```python
from build123d import *

# Parameters (mm, degrees)
BODY_DEPTH                     = 8
M3_CLEARANCE_SLOT1_DEPTH       = 8
LPATTERN3_COUNT                = 2
LPATTERN3_PITCH                = 31
LPATTERN3_COUNT_DIR2           = 2
LPATTERN3_PITCH_DIR2           = 31
CUT_EXTRUDE1_DEPTH             = 207.067949958
M3X0_5_TAPPED_HOLE1_D          = 2.5
LPATTERN2_COUNT                = 4
LPATTERN2_PITCH                = 25
CBORE_FOR_M5_SHCS1_D           = 5.5
CBORE_FOR_M5_SHCS1_CBORE_D     = 10
CBORE_FOR_M5_SHCS1_CBORE_DEPTH = 5
M3X0_5_TAPPED_HOLE2_D          = 2.5
M3X0_5_TAPPED_HOLE2_DEPTH      = 6.748924226
M3X0_5_TAPPED_HOLE2_TIP        = 0.751075774
SKETCH22_R                     = 2.5
CUT_EXTRUDE2_DEPTH             = 207.067949958


# Read off the part's stored shape, not the designer's step: M3 Clearance Slot1
with BuildPart() as part:
    # Sketch1 → BODY (new body)
    with BuildSketch(Plane.XY):
        with BuildLine():
            Line((-180, 100), (0, 100))
            Line((0, 100), (0, 0))
            Line((0, 0), (-50, 0))
            Line((-50, 0), (-50, 30))
            ThreePointArc((-50, 30), (-52.928932188, 37.071067812), (-60, 40))
            Line((-60, 40), (-180, 40))
            Line((-180, 40), (-180, 100))
        make_face()
    extrude(amount=BODY_DEPTH)

    # M3 Clearance Slot1 outline → M3 Clearance Slot1 (cut)
    with BuildSketch(Plane.XY):
        with BuildLine():
            Line((-42.3, 92.3), (-37.7, 92.3))
            ThreePointArc((-37.7, 92.3), (-36, 94), (-37.7, 95.7))
            Line((-37.7, 95.7), (-42.3, 95.7))
            ThreePointArc((-42.3, 95.7), (-44, 94), (-42.3, 92.3))
        make_face()
    m3_clearance_slot1 = extrude(amount=M3_CLEARANCE_SLOT1_DEPTH, mode=Mode.SUBTRACT)

    # LPattern3: M3 Clearance Slot1 2 × 2
    with Locations(*[(i * LPATTERN3_PITCH, -j * LPATTERN3_PITCH_DIR2, 0) for i in range(LPATTERN3_COUNT) for j in range(LPATTERN3_COUNT_DIR2) if (i, j) != (0, 0)]):
        add(m3_clearance_slot1, mode=Mode.SUBTRACT)

    # Sketch21 → Cut-Extrude1 (cut, through all)
    with BuildSketch(Plane.XY.offset(8)):
        with BuildLine():
            Line((-27, 89.5), (-22, 89.5))
            ThreePointArc((-22, 89.5), (-11, 78.5), (-22, 67.5))
            Line((-22, 67.5), (-27, 67.5))
            ThreePointArc((-27, 67.5), (-38, 78.5), (-27, 89.5))
        make_face()
    extrude(amount=-CUT_EXTRUDE1_DEPTH, mode=Mode.SUBTRACT)

    # M3x0.5 Tapped Hole1 (through all)
    with Locations(Plane.XY.offset(8)):
        with Locations((-70, 48)):
            m3x0_5_tapped_hole1 = Hole(M3X0_5_TAPPED_HOLE1_D / 2)

    # LPattern2: M3x0.5 Tapped Hole1 ×4
    with Locations(*[(-i * LPATTERN2_PITCH, 0, 0) for i in range(1, LPATTERN2_COUNT)]):
        add(m3x0_5_tapped_hole1, mode=Mode.SUBTRACT)

    # CBORE for M5 SHCS1 (through all)
    with Locations(Plane(origin=(0, 0, 0), x_dir=(-1, 0, 0), z_dir=(0, 0, -1))):
        with Locations((10, 6), (40, 6)):
            CounterBoreHole(CBORE_FOR_M5_SHCS1_D / 2, CBORE_FOR_M5_SHCS1_CBORE_D / 2, CBORE_FOR_M5_SHCS1_CBORE_DEPTH)

    # M3x0.5 Tapped Hole2
    with Locations(Plane.ZY.offset(180)):
        with Locations((4, 82), (4, 76)):
            Hole(M3X0_5_TAPPED_HOLE2_D / 2, depth=M3X0_5_TAPPED_HOLE2_DEPTH)
            with Locations((0, 0, -(M3X0_5_TAPPED_HOLE2_DEPTH + M3X0_5_TAPPED_HOLE2_TIP / 2))):  # 118° drill point
                Cone(0, M3X0_5_TAPPED_HOLE2_D / 2, M3X0_5_TAPPED_HOLE2_TIP, mode=Mode.SUBTRACT)

    # Sketch22 → Cut-Extrude2 (cut, through all)
    with BuildSketch(Plane.XY.offset(8)):
        with Locations((-170, 78.5)):
            Circle(SKETCH22_R)
    extrude(amount=-CUT_EXTRUDE2_DEPTH, mode=Mode.SUBTRACT)


solid = part.part
```
The model under review builds one solid part; all positions refer to its coordinate system, in mm. A direction names the side the tool comes from. Coordinates: 2 decimals unless noted, no trailing zeros. Write each loop counter-clockwise with the first axis right and the second up, starting at its lowest first coordinate (ties: lowest second). Pieces come first, ordered by that corner, then holes. Notation, with made-up numbers: (-13, -26) - (44, -26) arc R9 cw to (44, -15) - close; hole circle Ø4 at (-27, 28.25). An arc over 180 degrees is marked (long way). Answer in a Markdown table with one row per item. Add a question column.
Q1. To check wall thickness, follow line 1 along Y through (x, z) = (-170, 4.25); line 2 along Y through (x, z) = (-40, 3.15); line 3 along Y through (x, z) = (-43.5, 6.5). State the ranges of each line that lie inside material, in increasing order. Write a range as from..to.
Q2. Consider section A-A on y = 70. Give the boundary of the cut face in (x, z), then the cut area to 3 significant figures.
Q3. Draft analysis for pull direction Y (two halves, no side actions). For faces 1 (the face through (-119, 40, 4)), 2 (the face through (-89, 62, 0)), 3 (the face through (-40, 95.7, 4)), 4 (the face through (-5, 63, 4)), state which applies: +Y half, -Y half, draft (parallel to the pull), parting line (faces both ways), or undercut.
Q4. For faces 5 (the face through (-14.619, 4.085, 2.465)), 6 (the face through (-50, 15, 4)), 7 (the face through (-36, 94, 4)), list the 3-axis set-ups (+Z, -Z, +X, -X, +Y, -Y) from which the entire face can be reached by the end or side of a thin tool; tool diameter is ignored.
Q5. Clearance check with flat-ended pins moving along their axes: pin 1 (1.4 mm diameter, centred on x = -39.5, z = 5.5, fed in from -Y); pin 2 (2.5 mm diameter, centred on x = -138, z = 3.5, fed in from -Y); pin 3 (1.5 mm diameter, centred on x = -70, y = 48, fed in from +Z). State where each tip first meets the part, or that it passes through.
Q6. Consider section B-B on x = -128. Give the boundary of the cut face in (y, z), then the cut area to 3 significant figures.
Q7. Consider section C-C on y = 16.5. Give the boundary of the cut face in (x, z).
Answers below:
| question | item | result |
|---|---|---|
| 1 | line 1 | 40..76, 81..100 |
| 1 | line 2 | 0..1, 11..61.3, 64.7..92.3, 95.7..100 |
| 1 | line 3 | 0..61.8, 64.2..92.8, 95.2..100 |
| 2 | outline | (-180, 0) - (-33.98, 0) - (-33.98, 8) - (-180, 8) - close; (-15.02, 0) - (0, 0) - (0, 8) - (-15.02, 8) - close |
| 2 | area | 1,290 mm² |
| 3 | face 1 | -Y half |
| 3 | face 2 | draft |
| 3 | face 3 | undercut |
| 3 | face 4 | undercut |
| 4 | face 5 | -Z |
| 4 | face 6 | +Z, -Z, -X, -Y |
| 4 | face 7 | +Z, -Z |
| 5 | pin 1 | y = 0 |
| 5 | pin 2 | y = 40 |
| 5 | pin 3 | through |
| 6 | outline | (40, 0) - (100, 0) - (100, 8) - (40, 8) - close |
| 6 | area | 480 mm² |
| 7 | outline | (-50, 0) - (0, 0) - (0, 8) - (-50, 8) - close |
